```python
from build123d import *

# Parameters (mm, degrees)
SKETCH001_W  = 20
SKETCH001_H  = 20
PAD_DEPTH    = 3
SKETCH002_R  = 5.1
POCKET_DEPTH = 5


with BuildPart() as part:
    # Sketch001 → Pad (new body)
    with BuildSketch(Plane.XZ.offset(10)):
        with Locations((0, 10)):
            Rectangle(SKETCH001_W, SKETCH001_H)
    extrude(amount=PAD_DEPTH)

    # Sketch002 → Pocket (cut)
    with BuildSketch(Plane.XZ.offset(14)):
        with Locations((0, 10)):
            Circle(SKETCH002_R)
    extrude(amount=-POCKET_DEPTH, mode=Mode.SUBTRACT)


solid = part.part
```
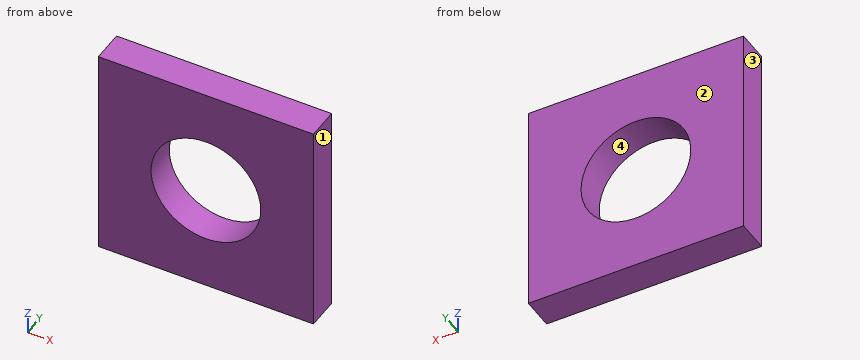
The model under review builds one solid part; all positions refer to its coordinate system, in mm. Face numbers are marked on the shaded views. Round coordinates to 2 decimals unless told otherwise and drop trailing zeros. Loops run counter-clockwise (first coordinate to the right, second up) from the corner with the lowest first, then second, coordinate; pieces in that order, holes last. Notation, with made-up numbers: M -14.75,53.5 L -2.75,53.5 A26 cw -2.75,76.5 Z; hole C 50,57 d9. An arc over 180 degrees is marked long. Put each result on its own line as item: value.
Q1. To check wall thickness, follow L1, parallel to Z at x = 0, y = -12.35; L2, parallel to X at y = -11.8, z = 6.25; L3, parallel to X at y = -10.7, z = 9.5. State the ranges of each line that lie inside material, in increasing order.
Result set:
L1: z = 0 to 4.9, 15.1 to 20
L2: x = -10 to -3.46, 3.46 to 10
L3: x = -10 to -5.08, 5.08 to 10
Q2. Consider section A-A, the plane x = 0. Give the boundary of the cut face in (y, z), then the cut area to 3 significant figures.
Result set:
outline: M -13,0 L -10,0 L -10,4.9 L -13,4.9 Z; M -13,15.1 L -10,15.1 L -10,20 L -13,20 Z
area: 29.4 mm²
Q3. Mouldability with a two-part tool opening along X and no side actions: class the marked faces 1, 2, 3 and 4 as released by +X, released by -X, zero draft, split by the parting line, or undercut.
Result set:
face 1: released by +X
face 2: zero draft
face 3: released by -X
face 4: undercut
Q4. Consider section B-B, the plane z = 10. Give the boundary of the cut face in (x, y).
Result set:
outline: M -10,-13 L -5.1,-13 L -5.1,-10 L -10,-10 Z; M 5.1,-13 L 10,-13 L 10,-10 L 5.1,-10 Z
Q5. Consider section C-C, the plane y = -10.5. Give the boundary of the cut face in (x, z).
Result set:
outline: M -10,0 L 10,0 L 10,20 L -10,20 Z; hole C 0,10 d10.2
